Here's how the part is built. I have some questions about the finished solid (model axes, mm). A direction names the side the tool comes from. Coordinates: 2 decimals unless noted, no trailing zeros. Loops run counter-clockwise (first coordinate to the right, second up) from the corner with the lowest first, then second, coordinate; pieces in that order, holes last. Notation, with made-up numbers: (75.5, 47.25) -> (131.5, 47.25) arc R15 ccw to (131.5, 58.25) -> close; hole circle Ø11 at (74.25, 34.5). An arc over 180 degrees is marked (long way). Answer as a JSON object with one key per item and string values. Group by question number.
Q1. I'm going to push flat-ended pins straight in: pin 1 (3 mm diameter, centred on x = -0.5, y = -6, fed in from +Z); pin 2 (1.5 mm diameter, centred on x = -1, z = -1, fed in from +Y); pin 3 (3.5 mm diameter, centred on y = -6, z = 0, fed in from +X); pin 4 (6 mm diameter, centred on y = -6.5, z = 8.5, fed in from +X). Where does each tip first touch, or does it pass through?
Q2. On a 3-axis mill with a long thin cutter (end or side, diameter ignored), from which of +Z, -Z, +X, -X, +Y, -Y can I reach the whole of each face in a straight line? I mean faces 4 (the flat face through (0, -5, -6)), 5 (the flat face through (-4.9, -3.8, -0.1)), 6 (the flat face through (0, -5, 6)), 7 (the flat face through (0, 4.78, 0)). Say none if no direction works.
Q3. I want a section at D-D on z = 10.5. Write out the boundary of the cut face in (x, y).
Q4. I need wall thicknesses on line 1 (Y direction, x = -2, z = 0); line 2 (X direction, y = 7.85, z = 0); line 3 (X direction, y = -3, z = 5.25). Which ranges of each line are inside material? Lowest first, please.
Q5. I want a section at C-C on y = -6. Write out the boundary of the cut face in (x, z), then the cut area to 3 significant figures.
Q6. Thinking about a two-plate mould opening in Z: for faces 1 (the cylindrical face through (2.52, 7.43, -0.33)), 2 (the flat face through (-1, 5, -12.5)), 3 (the flat face through (-1, 0, 8)), which applies, released by +Z, released by -Z, zero draft, split by the parting line, or undercut?
Q7. I want a section at B-B on z = 0. Write out the boundary of the cut face in (x, y).
Q8. I want a section at A-A on x = 4. Write out the boundary of the cut face in (y, z), then the cut area to 3 significant figures.
```python
from build123d import *

# Parameters (mm, degrees)
SKETCH1_W           = 99
SKETCH1_H           = 25
BOSS_EXTRUDE1_DEPTH = 10
SKETCH9_W           = 9.8
SKETCH9_H           = 12
BOSS_EXTRUDE9_DEPTH = 10
SKETCH10_R          = 2.54
CUT_EXTRUDE1_DEPTH  = 5.22
SKETCH11_R          = 2.05
CUT_EXTRUDE2_DEPTH  = 10


with BuildPart() as part:
    # Sketch1 → Boss-Extrude1 (new body)
    with BuildSketch(Plane(origin=(0, 0, 0), x_dir=(1, 0, 0), z_dir=(0, 1, 0))):
        Rectangle(SKETCH1_W, SKETCH1_H)
    extrude(amount=BOSS_EXTRUDE1_DEPTH)

    # Sketch9 → Boss-Extrude9 (add)
    with BuildSketch(Plane.XZ):
        Rectangle(SKETCH9_W, SKETCH9_H)
    extrude(amount=BOSS_EXTRUDE9_DEPTH)

    # Sketch10 → Cut-Extrude1 (cut)
    with BuildSketch(Plane(origin=(0, 10, 0), x_dir=(1, 0, 0), z_dir=(0, 1, 0))):
        with Locations(Location((0, 0, 0), (0, 0, 270))):
            Circle(SKETCH10_R)
    extrude(amount=-CUT_EXTRUDE1_DEPTH, mode=Mode.SUBTRACT)

    # Sketch11 → Cut-Extrude2 (cut)
    with BuildSketch(Plane(origin=(4.9, 0, 0), x_dir=(0, 0, -1), z_dir=(1, 0, 0))):
        with Locations((0, -6)):
            Circle(SKETCH11_R)
    extrude(amount=-CUT_EXTRUDE2_DEPTH, mode=Mode.SUBTRACT)


solid = part.part
```
Result set:
{
 "1": {"pin 1": "stops at z = 6", "pin 2": "stops at y = 4.78", "pin 3": "passes through", "pin 4": "stops at x = 4.9"},
 "2": {"face 4": "-Z, +X, -X, -Y", "face 5": "+Z, -Z, -X, -Y", "face 6": "+Z, +X, -X, -Y", "face 7": "+Y"},
 "3": {"outline": "(-49.5, 0) -> (49.5, 0) -> (49.5, 10) -> (-49.5, 10) -> close"},
 "4": {"line 1": "y = -10 to -8.05, -3.95 to 4.78", "line 2": "x = -49.5 to -2.54, 2.54 to 49.5", "line 3": "x = -4.9 to 4.9"},
 "5": {"outline": "(-4.9, -6) -> (4.9, -6) -> (4.9, -2.05) -> (-4.9, -2.05) -> close; (-4.9, 2.05) -> (4.9, 2.05) -> (4.9, 6) -> (-4.9, 6) -> close", "area": "77.4 mm²"},
 "6": {"face 1": "undercut", "face 2": "released by -Z", "face 3": "zero draft"},
 "7": {"outline": "(-49.5, 0) -> (-4.9, 0) -> (-4.9, -3.95) -> (4.9, -3.95) -> (4.9, 0) -> (49.5, 0) -> (49.5, 10) -> (2.54, 10) -> (2.54, 4.78) -> (-2.54, 4.78) -> (-2.54, 10) -> (-49.5, 10) -> close; (-4.9, -10) -> (4.9, -10) -> (4.9, -8.05) -> (-4.9, -8.05) -> close"},
 "8": {"outline": "(-10, -6) -> (0, -6) -> (0, -12.5) -> (10, -12.5) -> (10, 12.5) -> (0, 12.5) -> (0, 6) -> (-10, 6) -> close; hole circle Ø4.1 at (-6, 0)", "area": "357 mm²"}
}
